Can you work these out from the model? Positions are in its coordinate system, mm. A direction names the side the tool comes from. Give positions to 0.01 mm unless a question says otherwise; leave off trailing zeros. Order: outer loops, then holes, each group sorted by start corner. A loop starts at its lowest first (then second) coordinate and runs counter-clockwise, first axis right, second up. Notation, with made-up numbers: M 50.25,-25.75 L 100.25,-25.75 A30 cw 100.25,-3.75 Z; hole C 38.25,49.5 d9. An arc over 180 degrees is marked long. Use one line per item in the form item = value. Start each with the question number.
1. I want a section at A-A, the plane x = 0. List the corners of the cut face in (y, z) for me, and give its area (3 significant figures).
2. I want a section at D-D, the plane z = 0.75. List the corners of the cut face in (x, y) for me.
3. I want a section at B-B, the plane z = 2.5. List the corners of the cut face in (x, y) for me, and give its area (3 significant figures).
4. We'd pull the mould along X, two halves only. Please class faces 6 (the face through (6.466, 2.681, -2.465)), 7 (the face through (-6, 0, -3)), 8 (the face through (6, -2, -5)): +X half, -X half, draft (parallel to the pull), parting line (faces both ways), or undercut.
5. I need wall thicknesses on L1, parallel to X at y = 0, z = -2.5; L2, parallel to Y at x = 0, z = 5; L3, parallel to Z at x = 0.5, y = -3. Which ranges of each line are inside material? Lowest first, please.
6. Will these pins go through, and if not, where does the flat tip stop? P1, Ø1, axis at y = -4.5, z = 8.5, coming from the -X side; P2, Ø8, axis at x = 6, z = 4, coming from the -Y side; P3, Ø5, axis at x = 3.5, y = 0.5, coming from the +Z side.
7. I want a section at C-C, the plane y = 0. List the corners of the cut face in (x, z) for me, and give its area (3 significant figures).
8. For faces 1 (the face through (1.427, 9.48, 7.366)), 2 (the face through (-2.17, -9.76, 6.93)), 3 (the face through (-1.973, -8.884, 7.07)), 4 (the face through (-4.5, -8.1, 12)), 5 (the face through (0, 0, -1)), which set-ups out of +Z, -Z, +X, -X, +Y, -Y let a thin tool reach every point of the face, with its end or its side?
```python
from build123d import *

# Parameters (mm, degrees)
SKETCH_R        = 10
PAD_DEPTH       = 12
SKETCH001_R     = 9.1
POCKET_DEPTH    = 10
SKETCH002_R     = 7
PAD001_DEPTH    = 5
SKETCH003_R     = 6
POCKET001_DEPTH = 4
FILLET_R        = 2
SKETCH004_R     = 1.5
POCKET002_DEPTH = 11


with BuildPart() as part:
    # Sketch → Pad (new body)
    with BuildSketch(Plane.XY):
        Circle(SKETCH_R)
    extrude(amount=PAD_DEPTH)

    # Sketch001 (on Face3 of Pad) → Pocket (cut)
    with BuildSketch(Plane.XY.offset(12)):
        Circle(SKETCH001_R)
    extrude(amount=-POCKET_DEPTH, mode=Mode.SUBTRACT)

    # Sketch002 (on Face2 of Pocket) → Pad001 (join)
    with BuildSketch(Plane(origin=(0, 0, 0), x_dir=(1, 0, 0), z_dir=(0, 0, -1))):
        Circle(SKETCH002_R)
    extrude(amount=PAD001_DEPTH)

    # Sketch003 (on Face6 of Pad001) → Pocket001 (cut)
    with BuildSketch(Plane(origin=(0, 0, -5), x_dir=(1, 0, 0), z_dir=(0, 0, -1))):
        Circle(SKETCH003_R)
    extrude(amount=-POCKET001_DEPTH, mode=Mode.SUBTRACT)

    # Fillet
    fillet_edges = [part.edges().sort_by_distance(p)[0] for p in [
        (-10, 0, 0),
    ]]
    fillet(fillet_edges, radius=FILLET_R)

    # Sketch004 → Pocket002 (cut)
    with BuildSketch(Plane.XZ):
        with Locations((-0.003423, 6.915163)):
            Circle(SKETCH004_R)
    extrude(amount=-POCKET002_DEPTH, mode=Mode.SUBTRACT)


solid = part.part
```
Check result:
q1.outline = M -10,2 A2 ccw -8,0 L -7,0 L -7,-5 L -6,-5 L -6,-1 L 6,-1 L 6,-5 L 7,-5 L 7,0 L 8,0 A2 ccw 10,2 L 10,5.42 L 9.1,5.42 L 9.1,2 L -9.1,2 L -9.1,12 L -10,12 Z; M 9.1,8.42 L 10,8.42 L 10,12 L 9.1,12 Z
q1.area = 75.6 mm2
q2.outline = C 0,0 d19.12
q3.outline = C 0,0 d20; hole C 0,0 d18.2
q3.area = 54.0 mm2
q4.face_6 = parting line
q4.face_7 = undercut
q4.face_8 = draft
q5.L1 = -7 to -6, 6 to 7
q5.L2 = -10 to -9.1, 9.1 to 10
q5.L3 = -1 to 2
q6.P1 = -9.17
q6.P2 = -9.8
q6.P3 = 2
q7.outline = M -10,2 A2 ccw -8,0 L -7,0 L -7,-5 L -6,-5 L -6,-1 L 6,-1 L 6,-5 L 7,-5 L 7,0 L 8,0 A2 ccw 10,2 L 10,12 L 9.1,12 L 9.1,2 L -9.1,2 L -9.1,12 L -10,12 Z
q7.area = 78.3 mm2
q8.face_1 = +Y
q8.face_2 = +Z, -Z
q8.face_3 = +Z
q8.face_4 = +Z, +X, -X, +Y, -Y
q8.face_5 = -Z
